```python
from build123d import *


with BuildPart() as part:
    # Sweep2: sweep along a path in Sketch2
    with BuildLine(Plane(origin=(0, 0, 0), x_dir=(0, 0, -1), z_dir=(1, 0, 0))) as sweep2_path:
        Line((3.175, 0), (50.8, 0))
        Line((50.8, 0), (55.368806141, 2.22090307))
        ThreePointArc((55.368806141, 2.22090307), (59.019257676, -0.0635), (55.368806141, -2.34790307))
        Line((55.368806141, -2.34790307), (50.8, -0.127))
        Line((50.8, -0.127), (0, -0.127))
    # Sketch3 → Sweep2 (sweep)
    with BuildSketch(Plane.XY.offset(-3.175)):
        with BuildLine():
            Line((-1.5875, 0), (1.5875, 0))
            ThreePointArc((1.5875, 0), (0, 1.5875), (-1.5875, 0))
        make_face()
    sweep(path=sweep2_path.line, transition=Transition.RIGHT)


solid = part.part
```
Model file for the job. Use its own axes, mm. A direction names the side the tool comes from. Coordinates: 2 decimals unless noted, no trailing zeros. Loops run counter-clockwise (first coordinate to the right, second up) from the corner with the lowest first, then second, coordinate; pieces in that order, holes last. Notation, with made-up numbers: (78, 7) -> (127, 7) arc R26 ccw to (127, 39) -> close; hole circle Ø2 at (53.25, 39.25). An arc over 180 degrees is marked (long way). Answer as a JSON object with one key per item and string values.
Q1. Pull direction Z, two halves, no side cores. Call faces 1 (the cylindrical face through (-0.035, 2.553, -52.423)), 2 (the cylindrical face through (-0.035, 1.587, -27.321)), 3 (the flat face through (-0.02, -1.22, -53.05)): released by +Z, released by -Z, zero draft, split by the parting line, or undercut.
Report:
{"face 1": "released by +Z", "face 2": "zero draft", "face 3": "undercut"}
Q2. Cut at A-A (z = -18). List the corners of the cut face in (x, y) (1 decimal), and give its area (3 significant figures).
Report:
{"outline": "(-1.6, -0.1) arc R1.6 ccw to (1.6, -0.1) -> close; (-1.6, 0) -> (1.6, 0) arc R1.6 ccw to start", "area": "7.92 mm2"}
Q3. Cut at B-B (x = 0). List the corners of the cut face in (y, z) (1 decimal), and give its area (3 significant figures).
Report:
{"outline": "(-3.8, -54.7) arc R4.1 ccw (long way) to (3.6, -54.7) -> (1.6, -50.4) -> (1.6, -3.2) -> (0, -3.2) -> (0, -50.8) -> (2.2, -55.4) arc R2.5 cw (long way) to (-2.3, -55.4) -> (-0.1, -50.8) -> (-0.1, 0) -> (-1.7, 0) -> (-1.7, -50.4) -> close", "area": "193 mm2"}
Q4. Probe probe 1 along Z at (x, y) = (0, -1.75); probe 2 along X at (y, z) = (-0.25, -40.5); probe 3 along Y at (x, z) = (0.1, -53). List the from-to ranges inside material, lowest first.
Report:
{"probe 1": "z = -60.25 to -58.38, -54.14 to -50.51", "probe 2": "x = -1.58 to 1.58", "probe 3": "y = -2.96 to -1.2, 1.07 to 2.83"}
Q5. 3-axis set-ups, long thin cutter, end or side, ignore diameter. For faces 4 (the flat face through (-0.022, 1.126, -53.116)), 5 (the flat face through (0, -1, 0)), 6 (the flat face through (0, 1, -3.175)), 7 (the cylindrical face through (-0.035, -1.714, -25.044)): which of +Z, -Z, +X, -X, +Y, -Y reach the whole face in a straight line?
Report:
{"face 4": "+X, -X", "face 5": "+Z, +X, -X, +Y, -Y", "face 6": "+Z, +X, -X, +Y", "face 7": "+Z, -Y"}
Q6. Flat gauge pins, fed straight in: P1, Ø1.5, axis at y = -1, z = -21, coming from the +X side; P2, Ø1, axis at x = -0.5, z = -32.5, coming from the +Y side; P3, Ø1, axis at x = 1, y = 2, coming from the -Z side. Where does each tip first touch, or does it go through?
Report:
{"P1": "stops at x = 1.58", "P2": "stops at y = 1.59", "P3": "stops at z = -60.08"}
